Check sheet for the modelled part. Datum: model origin and axes. Units: mm. A direction names the side the tool comes from. Give positions to 0.01 mm unless a question says otherwise; leave off trailing zeros. Order: outer loops, then holes, each group sorted by start corner. A loop starts at its lowest first (then second) coordinate and runs counter-clockwise, first axis right, second up.
Item 1: Access from +Z, -Z, +X, -X, +Y, -Y to the whole of each face (thin tool, end or side, straight path). Record for faces 1 (the flat face through (46.228, 32, 8)), 2 (the flat face through (15.24, 32, 8)), 3 (the cylindrical face through (30.238, 35.655, 8.979)).
Item 2: Material ranges on line 1 along Z through (x, y) = (54.5, 6); line 2 along X through (y, z) = (39, 6.5), recorded low to high.
Item 3: Gauge pin test, flat ends, axial feed: P1, Ø7.5, axis at x = 29, z = 6, coming from the +Y side; P2, Ø6, axis at x = 30.734, y = 31.877, coming from the +Z side; P3, Ø4.5, axis at x = 27.5, z = 6, coming from the -Y side. Record the tip position at first contact, or that the pin passes through.
Item 4: Sectioned sample at C-C on z = 5. Record the boundary of the cut face in (x, y).
Item 5: Sectioned sample at D-D on x = 57.5. Record the boundary of the cut face in (y, z), and give its area (3 significant figures).
Item 6: Sectioned sample at A-A on x = 44. Record the boundary of the cut face in (y, z).
Item 7: Sectioned sample at B-B on y = 43.5. Record the boundary of the cut face in (x, z).
Item 8: Release check for a two-part mould opening along Y. For faces 4 (the flat face through (31, 24.638, 8)), 5 (the flat face through (31, 32, 2.54)), 6 (the flat face through (31, 36, 15.24)), 7 (the flat face through (31, 39.878, 8)) record: released by +Y, released by -Y, zero draft, split by the parting line, or undercut.
from build123d import *

# Parameters (mm, degrees)
F0_W     = 62.23
F0_H     = 63.5
F1_DEPTH = 44.45
F2_W     = 30.988
F2_H     = 15.24
F3_DEPTH = 15.24
F4_R     = 3.81
F5_DEPTH = 12.7


with BuildPart() as f1:
    # F0 (on Top) → F1 (new body)
    with BuildSketch(Plane.XY):
        with Locations((31.115, 31.75)):
            Rectangle(F0_W, F0_H)
    extrude(amount=-F1_DEPTH)

    # F2 (on face) → F3 (join)
    with BuildSketch(Plane.XY):
        with Locations((30.734, 32.258)):
            Rectangle(F2_W, F2_H)
    extrude(amount=F3_DEPTH)

    # F4 (on face) → F5 (cut)
    with BuildSketch(Plane.XY.offset(15.24)):
        with Locations((30.734, 31.877)):
            Circle(F4_R)
    extrude(amount=-F5_DEPTH, mode=Mode.SUBTRACT)


solid = f1.part
Report:
1. face 1: +Z, +X, +Y, -Y
1. face 2: +Z, -X, +Y, -Y
1. face 3: +Z
2. line 1: z = -44.45 to 0
2. line 2: x = 15.24 to 46.23
3. P1: stops at y = 39.88
3. P2: stops at z = 2.54
3. P3: stops at y = 24.64
4. outline: (15.24, 24.64) - (46.23, 24.64) - (46.23, 39.88) - (15.24, 39.88) - close; hole circle Ø7.62 at (30.73, 31.88)
5. outline: (0, -44.45) - (63.5, -44.45) - (63.5, 0) - (0, 0) - close
5. area: 2,820 mm2
6. outline: (0, -44.45) - (63.5, -44.45) - (63.5, 0) - (39.88, 0) - (39.88, 15.24) - (24.64, 15.24) - (24.64, 0) - (0, 0) - close
7. outline: (0, -44.45) - (62.23, -44.45) - (62.23, 0) - (0, 0) - close
8. face 4: released by -Y
8. face 5: undercut
8. face 6: zero draft
8. face 7: released by +Y
